```python
from build123d import *

# Parameters (mm, degrees)
F0_R     = 250
F0_R_2   = 12.05
F1_DEPTH = 20
F2_R     = 7.5
F3_DEPTH = 20
F4_R     = 12.5
F5_DEPTH = 20


with BuildPart() as f1:
    # F0 (on Top) → F1 (new body)
    with BuildSketch(Plane.XY):
        Circle(F0_R)
        Circle(F0_R_2, mode=Mode.SUBTRACT)
    extrude(amount=F1_DEPTH)

    # F2 (on face) → F3 (cut, through all)
    with BuildSketch(Plane.XY.offset(20)):
        with Locations((219.748125, 58.881333)):
            Circle(F2_R)
        with Locations((160.866793, 160.866793)):
            Circle(F2_R)
        with Locations((58.881333, 219.748125)):
            Circle(F2_R)
        with Locations((-58.881333, 219.748125)):
            Circle(F2_R)
        with Locations((-160.866793, 160.866793)):
            Circle(F2_R)
        with Locations((-219.748125, 58.881333)):
            Circle(F2_R)
        with Locations((-219.748125, -58.881333)):
            Circle(F2_R)
        with Locations((-160.866793, -160.866793)):
            Circle(F2_R)
        with Locations((-58.881333, -219.748125)):
            Circle(F2_R)
        with Locations((58.881333, -219.748125)):
            Circle(F2_R)
        with Locations((160.866793, -160.866793)):
            Circle(F2_R)
        with Locations((219.748125, -58.881333)):
            Circle(F2_R)
    extrude(amount=-F3_DEPTH, mode=Mode.SUBTRACT)

    # F4 (on face) → F5 (cut)
    with BuildSketch(Plane.XY.offset(20)):
        with Locations((186.35709, 130.488639)):
            Circle(F4_R)
        with Locations((-186.35709, 130.488639)):
            Circle(F4_R)
        with Locations((-186.35709, -130.488639)):
            Circle(F4_R)
        with Locations((186.35709, -130.488639)):
            Circle(F4_R)
    extrude(amount=-F5_DEPTH, mode=Mode.SUBTRACT)


solid = f1.part
```
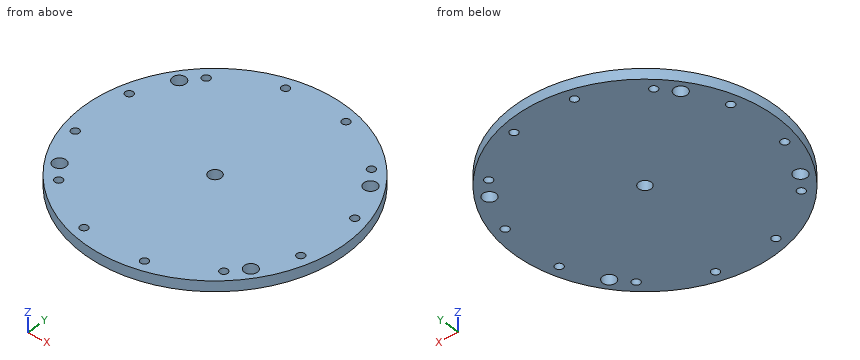
Verification items for the finished model (mm, model axes). Coordinates: 2 decimals unless noted, no trailing zeros. Write each loop counter-clockwise with the first axis right and the second up, starting at its lowest first coordinate (ties: lowest second). Pieces come first, ordered by that corner, then holes. Notation, with made-up numbers: M 64,-13.75 L 106,-13.75 A23 ccw 106,13.25 Z; hole C -6.5,-16.75 d4. An arc over 180 degrees is marked long. Answer as a JSON object with one key per item and string values. Group by question number.
(1) Cross-section at C-C, the plane z = 3.5. State how many separate pieces and enclosed holes the cut face has, and give its area (3 significant figures).
(2) Cross-section at D-D, the plane x = -184.5. Record the cut outline in (y, z).
(3) Material ranges on line 1 (Y direction, x = -187.5, z = 6.5); line 2 (Y direction, x = -224, z = 4.25); line 3 (X direction, y = -137, z = 1.75), recorded low to high.
(4) Gauge pin test, flat ends, axial feed: pin 1 (24 mm diameter, centred on x = 219.75, y = -58.88, fed in from +Z); pin 2 (10 mm diameter, centred on x = -28.5, z = 10.5, fed in from +Y); pin 3 (2 mm diameter, centred on x = 89, z = 7, fed in from +Y); pin 4 (10 mm diameter, centred on x = 75.5, z = 15, fed in from -Y). Record the tip position at first contact, or that the pin passes through.
(5) Cross-section at A-A, the plane y = 0. Record the cut outline in (x, z).
Reply:
{
 "1": {"separate pieces": "1", "enclosed holes": "17", "area": "192,000 mm²"},
 "2": {"outline": "M -168.7,0 L -142.85,0 L -142.85,20 L -168.7,20 Z; M -118.13,0 L 118.13,0 L 118.13,20 L -118.13,20 Z; M 142.85,0 L 168.7,0 L 168.7,20 L 142.85,20 Z"},
 "3": {"line 1": "-165.36 to -142.94, -118.04 to 118.04, 142.94 to 165.36", "line 2": "-111.01 to -65.06, -52.7 to 52.7, 65.06 to 111.01", "line 3": "-209.12 to -197.03, -175.69 to 175.69, 197.03 to 209.12"},
 "4": {"pin 1": "z = 20", "pin 2": "y = 248.89", "pin 3": "y = 234", "pin 4": "y = -239.85"},
 "5": {"outline": "M -250,0 L -12.05,0 L -12.05,20 L -250,20 Z; M 12.05,0 L 250,0 L 250,20 L 12.05,20 Z"}
}
